Geometry: see drawing. Coordinates: mm, zero at the bounding-box minimum. A direction names the side the tool comes from. Coordinates: 2 decimals unless noted, no trailing zeros. Write each loop counter-clockwise with the first axis right and the second up, starting at its lowest first coordinate (ties: lowest second). Pieces come first, ordered by that corner, then holes.
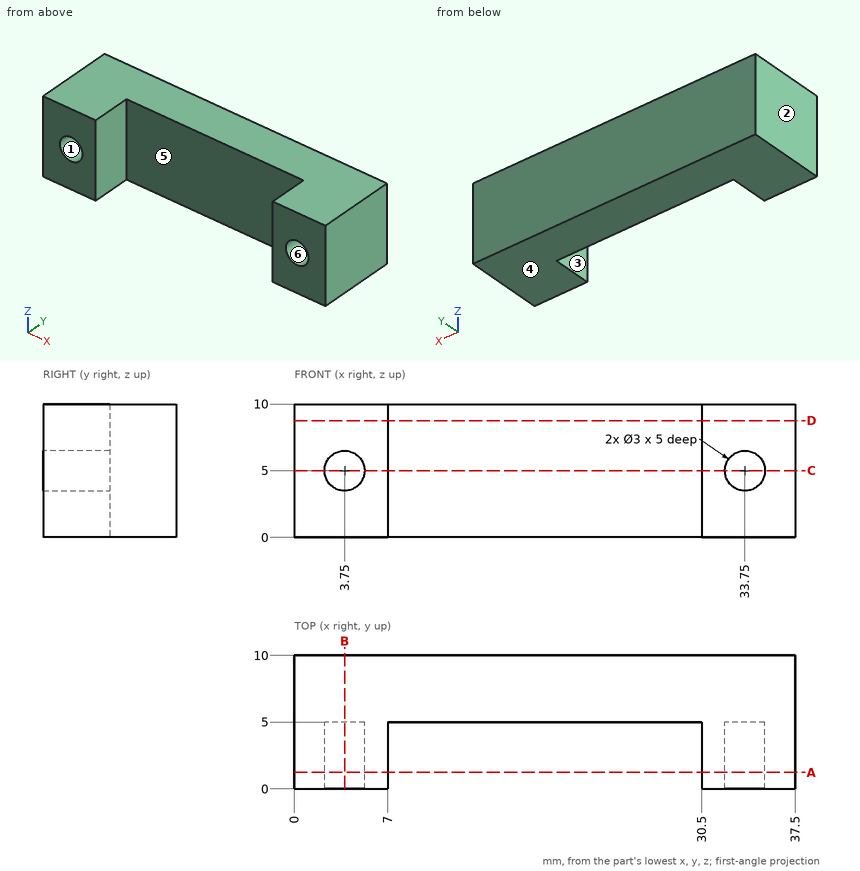
Item 1: Set-up query: the marked faces 1, 2 and 3. Return all of +Z, -Z, +X, -X, +Y, -Y with unobstructed straight access to the full face (end or side cutting, diameter ignored); none if empty.
Derived:
face 1: -Y
face 2: +Z, -Z, -X, +Y, -Y
face 3: +Z, -Z, -Y
Item 2: Section D-D, the plane z = 8.75. Output: boundary loops of the cut face in (x, y).
Derived:
outline: (0, 0) - (7, 0) - (7, 5) - (30.5, 5) - (30.5, 0) - (37.5, 0) - (37.5, 10) - (0, 10) - close
Item 3: Pin query (flat end, axial travel): pin 1 (0.9 mm diameter, centred on x = 4, z = 4.5, fed in from -Y). Return the tip coordinate at first contact, or that it passes through.
Derived:
pin 1: stops at y = 5
Item 4: Section A-A, the plane y = 1.25. Output: boundary loops of the cut face in (x, z).
Derived:
outline: (0, 0) - (7, 0) - (7, 10) - (0, 10) - close; (30.5, 0) - (37.5, 0) - (37.5, 10) - (30.5, 10) - close; hole circle Ø3 at (3.75, 5); hole circle Ø3 at (33.75, 5)
Item 5: Section C-C, the plane z = 5. Output: boundary loops of the cut face in (x, y).
Derived:
outline: (0, 0) - (2.25, 0) - (2.25, 5) - (5.25, 5) - (5.25, 0) - (7, 0) - (7, 5) - (30.5, 5) - (30.5, 0) - (32.25, 0) - (32.25, 5) - (35.25, 5) - (35.25, 0) - (37.5, 0) - (37.5, 10) - (0, 10) - close
Item 6: Section B-B, the plane x = 3.75. Output: boundary loops of the cut face in (y, z), plus the area to 3 significant figures.
Derived:
outline: (0, 0) - (10, 0) - (10, 10) - (0, 10) - (0, 6.5) - (5, 6.5) - (5, 3.5) - (0, 3.5) - close
area: 85.0 mm2
Item 7: Material intervals for probe 1 along X at (y, z) = (3.85, 5); probe 2 along X at (y, z) = (1.5, 8); probe 3 along Y at (x, z) = (15, 5), sorted ascending.
Derived:
probe 1: x = 0 to 2.25, 5.25 to 7, 30.5 to 32.25, 35.25 to 37.5
probe 2: x = 0 to 7, 30.5 to 37.5
probe 3: y = 5 to 10
Item 8: Pull-direction query (Z, two-part tool) for the marked faces 4, 5 and 6; classes: released by +Z, released by -Z, zero draft, split by the parting line, or undercut.
Derived:
face 4: released by -Z
face 5: zero draft
face 6: undercut
